For this review, take the finished solid that the model builds, in its own axes (mm). Face numbers are marked on the shaded views. A direction names the side the tool comes from. Round coordinates to 2 decimals unless told otherwise and drop trailing zeros. Order: outer loops, then holes, each group sorted by start corner. A loop starts at its lowest first (then second) coordinate and runs counter-clockwise, first axis right, second up. Notation, with made-up numbers: (39, 53.25) -> (45, 53.25) arc R24 ccw to (45, 91.25) -> close; hole circle Ø3 at (21, 76.25). An arc over 180 degrees is marked (long way). Answer in a Markdown table with one row per item.
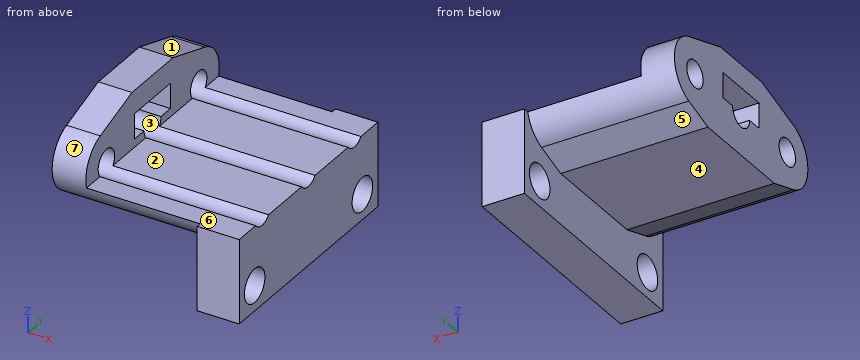
```python
from build123d import *

# Parameters (mm, degrees)
ESBO_O1_W                     = 5
ESBO_O1_H                     = 27
RESSALTO_EXTRUS_O1_DEPTH      = 4
RESSALTO_EXTRUS_O1_DEPTH_BACK = 6
ESBO_O2_W                     = 4
ESBO_O2_H                     = 27
RESSALTO_EXTRUS_O2_DEPTH      = 17.5
ESBO_O3_W                     = 4
ESBO_O3_H                     = 27
RESSALTO_EXTRUS_O3_DEPTH      = 6.75232
CORTE_EXTRUS_O1_DEPTH         = 17.5
ESBO_O5_R                     = 1.598160281
ESBO_O5_R_2                   = 1.600993429
CORTE_EXTRUS_O2_DEPTH         = 23.5
ESBO_O6_R                     = 2
CORTE_EXTRUS_O3_DEPTH         = 14


with BuildPart() as part:
    # Esboço1 → Ressalto-extrusão1 (new body, two sides)
    with BuildSketch(Plane.XY) as ressalto_extrus_o1_sk:
        with Locations((2.5, 202.468429513)):
            Rectangle(ESBO_O1_W, ESBO_O1_H)
    extrude(amount=RESSALTO_EXTRUS_O1_DEPTH)
    extrude(ressalto_extrus_o1_sk.sketch, amount=-RESSALTO_EXTRUS_O1_DEPTH_BACK)

    # Esboço2 → Ressalto-extrusão2 (add)
    with BuildSketch(Plane.ZY):
        with Locations((2, 202.468429513)):
            Rectangle(ESBO_O2_W, ESBO_O2_H)
    extrude(amount=RESSALTO_EXTRUS_O2_DEPTH)

    # Esboço3 → Ressalto-extrusão3 (add)
    with BuildSketch(Plane.XY.offset(4)):
        with Locations((-15.5, 202.468429513)):
            Rectangle(ESBO_O3_W, ESBO_O3_H)
    extrude(amount=RESSALTO_EXTRUS_O3_DEPTH)

    # Esboço4 → Corte-extrusão1 (cut)
    with BuildSketch(Plane.ZY.offset(17.5)):
        with BuildLine():
            Line((10.752320108, 206.42333876), (10.752320108, 215.968429513))
            Line((10.752320108, 215.968429513), (0, 215.968429513))
            Line((0, 215.968429513), (0, 208.891636686))
            Line((0, 208.891636686), (1.172017461, 212.62112057))
            ThreePointArc((1.172017461, 212.62112057), (4.990885368, 215.423316276), (8.808422699, 212.619308145))
            Line((8.808422699, 212.619308145), (10.752320108, 206.42333876))
        make_face()
        with BuildLine():
            Line((10.752320108, 198.42333838), (10.752320108, 188.968429513))
            Line((10.752320108, 188.968429513), (0, 188.968429513))
            Line((0, 188.968429513), (0, 195.95406786))
            Line((0, 195.95406786), (1.171653646, 192.22427259))
            ThreePointArc((1.171653646, 192.22427259), (4.988209463, 189.422715847), (8.804822441, 192.224194718))
            Line((8.804822441, 192.224194718), (10.752320108, 198.42333838))
        make_face()
    extrude(amount=-CORTE_EXTRUS_O1_DEPTH, mode=Mode.SUBTRACT)

    # Esboço5 → Corte-extrusão2 (cut, through all)
    with BuildSketch(Plane.ZY.offset(17.5)):
        with Locations((4.989935533, 211.421312021)):
            Circle(ESBO_O5_R)
        with Locations((4.988250275, 193.423193451)):
            Circle(ESBO_O5_R_2)
        with BuildLine():
            Line((4.9893193, 200.772419725), (4.9893193, 198.92333857))
            Line((4.9893193, 198.92333857), (7.9893193, 198.92333857))
            Line((7.9893193, 198.92333857), (7.9893193, 205.92333857))
            Line((7.9893193, 205.92333857), (4.9893193, 205.92333857))
            Line((4.9893193, 205.92333857), (4.9893193, 204.074257415))
            ThreePointArc((4.9893193, 204.074257415), (3.338400455, 202.42333857), (4.9893193, 200.772419725))
        make_face()
    extrude(amount=-CORTE_EXTRUS_O2_DEPTH, mode=Mode.SUBTRACT)

    # Esboço6 → Corte-extrusão3 (cut)
    with BuildSketch(Plane.ZY):
        with Locations((-3, 212.968429513)):
            Circle(ESBO_O6_R)
        with Locations((-3, 191.968429513)):
            Circle(ESBO_O6_R)
    extrude(amount=-CORTE_EXTRUS_O3_DEPTH, mode=Mode.SUBTRACT)


solid = part.part
```
Q1. Tool access review of the marked faces 4, 5, 6 and 7: name each direction out of +Z, -Z, +X, -X, +Y, -Y from which nothing blocks a thin tool from reaching the whole face with its end or side.
Answer key:
| item | result |
|---|---|
| face 4 | -Z, -X, +Y, -Y |
| face 5 | -Z, -X, +Y |
| face 6 | +Z, +X, +Y, -Y |
| face 7 | -X, -Y |
Q2. Take a section at B-B, the plane z = 7.25. Write out the cut boundary in (x, y).
Answer key:
| item | result |
|---|---|
| outline | (-17.5, 190.12) -> (-13.5, 190.12) -> (-13.5, 198.92) -> (-17.5, 198.92) -> close; (-17.5, 205.92) -> (-13.5, 205.92) -> (-13.5, 214.72) -> (-17.5, 214.72) -> close |
Q3. Take a section at D-D, the plane x = 1. Write out the cut boundary in (y, z) (3 decimals), then the cut area to 3 significant figures.
Answer key:
| item | result |
|---|---|
| outline | (188.968, -6) -> (215.968, -6) -> (215.968, 4) -> (212.676, 4) arc R1.598 cw to (210.167, 4) -> (203.745, 4) arc R1.651 cw to (201.102, 4) -> (194.683, 4) arc R1.601 cw to (192.164, 4) -> (188.968, 4) -> close; hole circle Ø4 at (191.968, -3); hole circle Ø4 at (212.968, -3) |
| area | 242 mm^2 |
Q4. Clearance check with flat-ended pins moving along their axes: pin 1 Ø10 at (x, z) = (-9, 4.5) entering from -Y; pin 2 Ø3 at (x, y) = (-16, 201) entering from -Z; pin 3 Ø2 at (y, z) = (197, 7) entering from +X. State where each tip first meets the part, or that it passes through.
Answer key:
| item | result |
|---|---|
| pin 1 | stops at y = 189.42 |
| pin 2 | stops at z = 0 |
| pin 3 | stops at x = -13.5 |
Q5. The part is to be moulded in two halves that separate along Y. For the marked faces 1, 2 and 3, say which applies: +Y half, -Y half, draft (parallel to the pull), parting line (faces both ways), or undercut.
Answer key:
| item | result |
|---|---|
| face 1 | +Y half |
| face 2 | draft |
| face 3 | undercut |
Q6. To check wall thickness, follow probe 1 along Y at (x, z) = (2.9, -3); probe 2 along Z at (x, y) = (2.5, 192); probe 3 along X at (y, z) = (212.5, 0.75). State the ranges of each line that lie inside material, in increasing order.
Answer key:
| item | result |
|---|---|
| probe 1 | y = 188.97 to 189.97, 193.97 to 210.97, 214.97 to 215.97 |
| probe 2 | z = -6 to -5, -1 to 4 |
| probe 3 | x = 0 to 5 |
Q7. Take a section at C-C, the plane x = -15. Write out the cut boundary in (y, z), then the cut area to 3 significant figures.
Answer key:
| item | result |
|---|---|
| outline | (192.22, 1.17) -> (195.95, 0) -> (208.89, 0) -> (212.62, 1.17) arc R4 ccw to (212.62, 8.81) -> (206.42, 10.75) -> (198.42, 10.75) -> (192.22, 8.8) arc R4 ccw to start; hole circle Ø3.2 at (193.42, 4.99); hole (198.92, 4.99) -> (200.77, 4.99) arc R1.65 ccw to (204.07, 4.99) -> (205.92, 4.99) -> (205.92, 7.99) -> (198.92, 7.99) -> close; hole circle Ø3.2 at (211.42, 4.99) |
| area | 193 mm^2 |
Q8. Take a section at A-A, the plane z = -3. Write out the cut boundary in (x, y).
Answer key:
| item | result |
|---|---|
| outline | (0, 188.97) -> (5, 188.97) -> (5, 189.97) -> (0, 189.97) -> close; (0, 193.97) -> (5, 193.97) -> (5, 210.97) -> (0, 210.97) -> close; (0, 214.97) -> (5, 214.97) -> (5, 215.97) -> (0, 215.97) -> close |
